```python
from build123d import *

# Parameters (mm, degrees)
SKETCH1_R           = 1.5
SKETCH1_W           = 20.26
SKETCH1_H           = 3
BOSS_EXTRUDE1_DEPTH = 3


with BuildPart() as part:
    # Sketch1 → Boss-Extrude1 (new body)
    with BuildSketch(Plane(origin=(0, 0, 0), x_dir=(1, 0, 0), z_dir=(0, 1, 0))):
        Polygon((-5, 0), (5, 0), (5, 3), (14, 3), (14, 25), (-14, 25), (-14, 3), (-5, 3), align=None)
        with Locations(Location((7.63, 19.1, 0), (0, 0, 270))):
            Circle(SKETCH1_R, mode=Mode.SUBTRACT)
        with Locations(Location((-7.63, 19.1, 0), (0, 0, 90))):
            Circle(SKETCH1_R, mode=Mode.SUBTRACT)
        with Locations((0, 7.7)):
            Rectangle(SKETCH1_W, SKETCH1_H, mode=Mode.SUBTRACT)
    extrude(amount=BOSS_EXTRUDE1_DEPTH)


solid = part.part
```
Model file for the job. Use its own axes, mm. A direction names the side the tool comes from. Coordinates: 2 decimals unless noted, no trailing zeros. Loops run counter-clockwise (first coordinate to the right, second up) from the corner with the lowest first, then second, coordinate; pieces in that order, holes last. Notation, with made-up numbers: (-18, -25) - (22, -25) arc R19 cw to (22, 6) - close; hole circle Ø4 at (-33.75, -24). An arc over 180 degrees is marked (long way). Write item = value, one per line. Start each with the question number.
Item 1: Saw through at C-C, the plane z = -19.1. List the corners of the cut face in (x, y), then the cut area to 3 significant figures.
Item 2: Saw through at A-A, the plane x = 7.63. List the corners of the cut face in (y, z), then the cut area to 3 significant figures.
Item 3: Saw through at B-B, the plane y = 0.75. List the corners of the cut face in (x, z), then the cut area to 3 significant figures.
Item 4: Pull direction X, two halves, no side cores. Call faces 1 (the face through (14, 1, -14)), 2 (the face through (0, 1, 0)), 3 (the face through (0, 1, -9.2)): +X half, -X half, draft (parallel to the pull), parting line (faces both ways), or undercut.
Item 5: Saw through at D-D, the plane x = 3.5. List the corners of the cut face in (y, z).
Item 6: Drop flat-ended pins along their axis: pin 1 Ø2.5 at (x, z) = (-7.63, -19.1) entering from -Y; pin 2 Ø1.5 at (x, y) = (10.5, 1.5) entering from +Z. Give the stop position or say it passes through.
Item 7: Wall check: probe 1 along X at (y, z) = (1.4, -19.1); probe 2 along Z at (x, y) = (-7.63, 1.7); probe 3 along Z at (x, y) = (2, 1.6). Give the ranges that are in metal, low to high. Write a range as [from, to].
Item 8: 3-axis set-ups, long thin cutter, end or side, ignore diameter. For faces 4 (the face through (0, 1, -25)), 5 (the face through (10.13, 1, -8)), 6 (the face through (5, 1, -1)), 7 (the face through (-10, 1, -3)), 8 (the face through (0, 0, -15)): which of +Z, -Z, +X, -X, +Y, -Y reach the whole face in a straight line?
Answers:
q1.outline = (-14, 0) - (-9.13, 0) - (-9.13, 3) - (-14, 3) - close; (-6.13, 0) - (6.13, 0) - (6.13, 3) - (-6.13, 3) - close; (9.13, 0) - (14, 0) - (14, 3) - (9.13, 3) - close
q1.area = 66.0 mm2
q2.outline = (0, -25) - (3, -25) - (3, -20.6) - (0, -20.6) - close; (0, -17.6) - (3, -17.6) - (3, -9.2) - (0, -9.2) - close; (0, -6.2) - (3, -6.2) - (3, -3) - (0, -3) - close
q2.area = 48.0 mm2
q3.outline = (-14, -25) - (14, -25) - (14, -3) - (5, -3) - (5, 0) - (-5, 0) - (-5, -3) - (-14, -3) - close; hole (-10.13, -9.2) - (10.13, -9.2) - (10.13, -6.2) - (-10.13, -6.2) - close; hole circle Ø3 at (-7.63, -19.1); hole circle Ø3 at (7.63, -19.1)
q3.area = 571 mm2
q4.face_1 = +X half
q4.face_2 = draft
q4.face_3 = undercut
q5.outline = (0, -25) - (3, -25) - (3, -9.2) - (0, -9.2) - close; (0, -6.2) - (3, -6.2) - (3, 0) - (0, 0) - close
q6.pin_1 = through
q6.pin_2 = -3
q7.probe_1 = [-14, -9.13], [-6.13, 6.13], [9.13, 14]
q7.probe_2 = [-25, -20.6], [-17.6, -9.2], [-6.2, -3]
q7.probe_3 = [-25, -9.2], [-6.2, 0]
q8.face_4 = -Z, +X, -X, +Y, -Y
q8.face_5 = +Y, -Y
q8.face_6 = +Z, +X, +Y, -Y
q8.face_7 = +Z, -X, +Y, -Y
q8.face_8 = +Z, -Z, +X, -X, -Y
